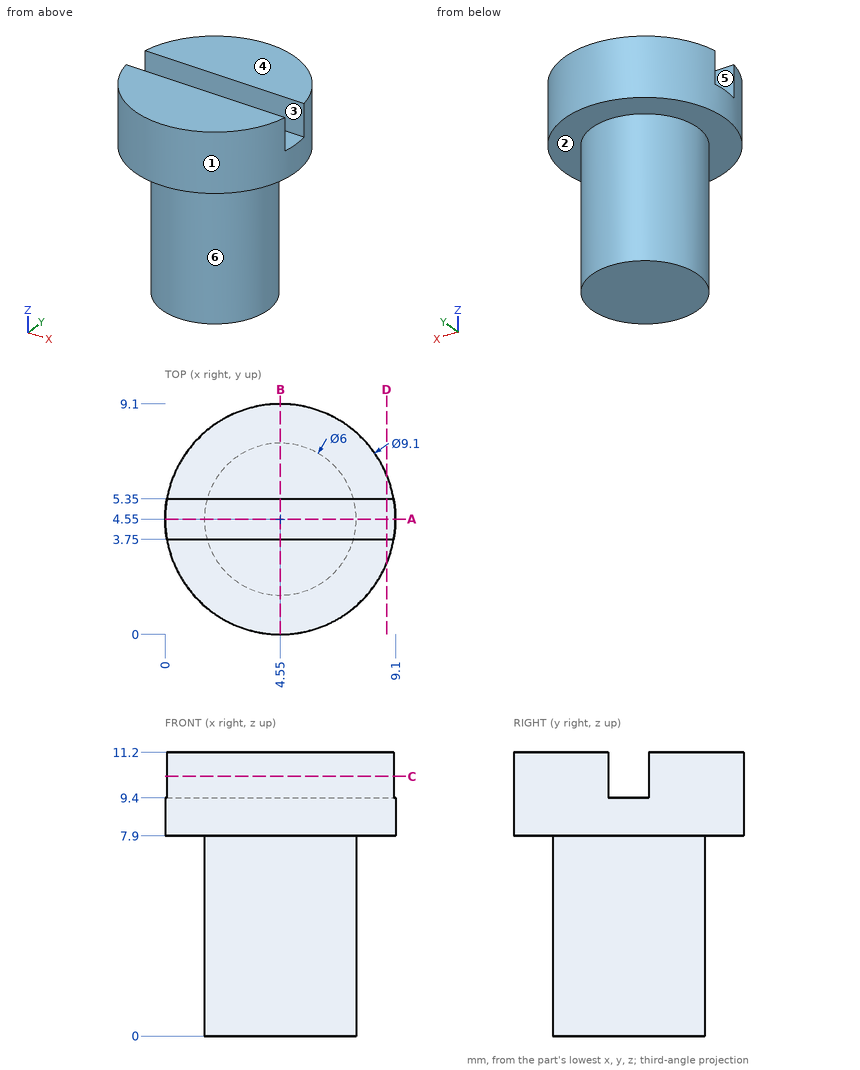
Study the drawing (mm; zero at the part's minimum x, y, z) and answer. A direction names the side the tool comes from. Round coordinates to 2 decimals unless told otherwise and drop trailing zeros. Loops run counter-clockwise (first coordinate to the right, second up) from the corner with the lowest first, then second, coordinate; pieces in that order, holes last.
Q1. Section C-C, the plane z = 10.25 is taken. Determine the outline of the cut face in (x, y), then the cut area to 3 significant figures.
Q2. Find the intervals of material crossed by line 1 (Z direction, x = 1, y = 6); line 2 (Z direction, x = 8.5, y = 5.25); line 3 (X direction, y = 4.5, z = 4.5), in increasing order.
Q3. Section B-B, the plane x = 4.55 is taken. Determine the outline of the cut face in (y, z).
Q4. Section D-D, the plane x = 8.75 is taken. Determine the outline of the cut face in (y, z).
Q5. Given pin 1 Ø0.5 at (x, z) = (3, 10.5) entering from +Y; pin 2 Ø5 at (y, z) = (5.5, 4) entering from +X; pin 3 Ø3 at (x, z) = (3, 2) entering from +Y, each flat-ended and moving along its own axis, determine where each tip first touches the part or whether it passes through.
Q6. For a pull along Y with two mould halves and no side action, classify the marked faces 4, 5 and 6 as released by +Y, released by -Y, zero draft, split by the parting line, or undercut.
Q7. Section A-A, the plane y = 4.55 is taken. Determine the outline of the cut face in (x, z), then the cut area to 4 significant figures.
Q8. Which of the six approach directions +Z, -Z, +X, -X, +Y, -Y give full straight-line access (tool end or side, diameter ignored) to the marked faces 1, 2 and 3?
Completed:
1. outline: (0.07, 3.75) arc R4.55 ccw to (9.03, 3.75) - close; (0.07, 5.35) - (9.03, 5.35) arc R4.55 ccw to start
1. area: 50.6 mm2
2. line 1: z = 7.9 to 11.2
2. line 2: z = 7.9 to 9.4
2. line 3: x = 1.55 to 7.55
3. outline: (0, 7.9) - (1.55, 7.9) - (1.55, 0) - (7.55, 0) - (7.55, 7.9) - (9.1, 7.9) - (9.1, 11.2) - (5.35, 11.2) - (5.35, 9.4) - (3.75, 9.4) - (3.75, 11.2) - (0, 11.2) - close
4. outline: (2.8, 7.9) - (6.3, 7.9) - (6.3, 11.2) - (5.35, 11.2) - (5.35, 9.4) - (3.75, 9.4) - (3.75, 11.2) - (2.8, 11.2) - close
5. pin 1: stops at y = 8.91
5. pin 2: stops at x = 7.55
5. pin 3: stops at y = 7.55
6. face 4: zero draft
6. face 5: undercut
6. face 6: split by the parting line
7. outline: (0, 7.9) - (1.55, 7.9) - (1.55, 0) - (7.55, 0) - (7.55, 7.9) - (9.1, 7.9) - (9.1, 9.4) - (0, 9.4) - close
7. area: 61.05 mm2
8. face 1: +Z, -Z
8. face 2: -Z
8. face 3: +Z, +X, -X
